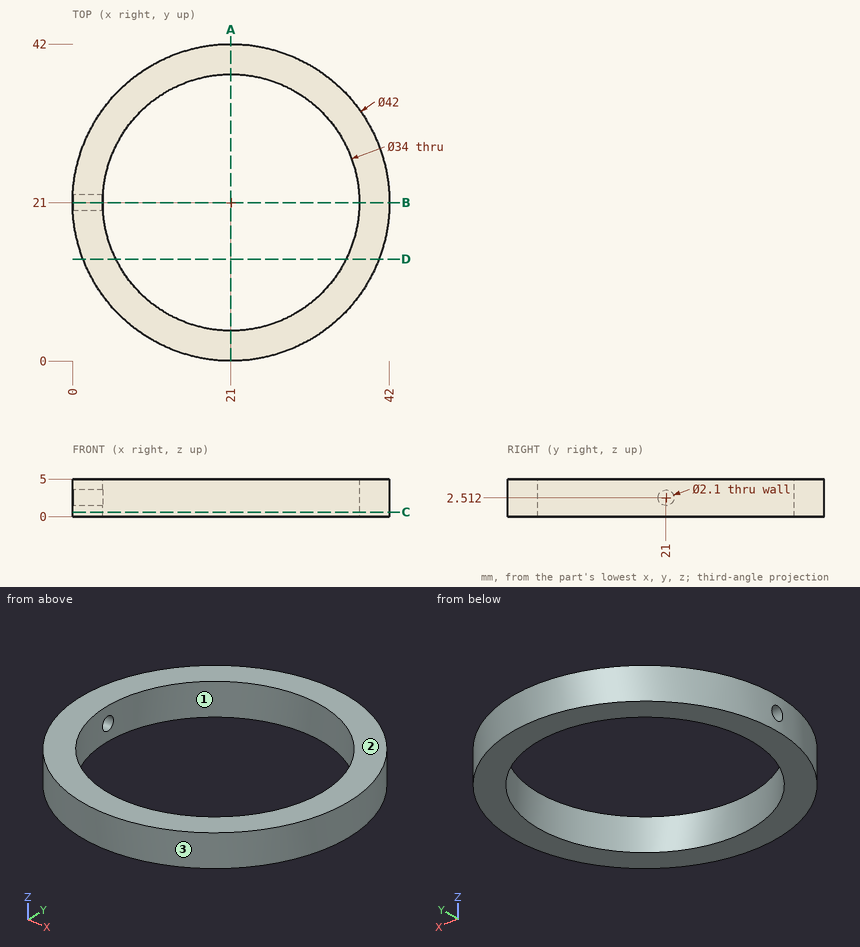
Design review of the part shown in the three views and the two pictorial views. Dimensions are in mm from the part's minimum x, y and z. Round coordinates to 2 decimals unless told otherwise and drop trailing zeros. Write each loop counter-clockwise with the first axis right and the second up, starting at its lowest first coordinate (ties: lowest second). Pieces come first, ordered by that corner, then holes. Notation, with made-up numbers: (2, 10.25) -> (38, 10.25) arc R11 ccw to (38, 17.25) -> close; hole circle Ø9 at (66.5, 83.5). An arc over 180 degrees is marked (long way). One line per question, with ' | ' between items. Start each with the question number.
1) Add section B-B (y = 21). Write out the cut boundary in (x, z).
2) For pin 1 Ø2.5 at (y, z) = (21, 2.51) entering from -X; pin 2 Ø2 at (y, z) = (34.5, 4) entering from -X (1 decimal); pin 3 Ø2 at (x, z) = (31.5, 0.5) entering from +Y, all flat-tipped, find the tip position at first contact; note any pin that passes through.
3) Add section A-A (x = 21). Write out the cut boundary in (y, z).
4) Wall thickness on line 1 along Y through (x, z) = (21, 3.55); line 2 along X through (y, z) = (31.5, 4.35); line 3 along Y through (x, z) = (18, 4.5) (1 decimal): over which ranges is each line inside the solid? List them lowest first.
5) Add section C-C (z = 0.6). Write out the cut boundary in (x, y).
6) Add section D-D (y = 13.5). Write out the cut boundary in (x, z) (3 decimals).
7) Mouldability with a two-part tool opening along Y and no side actions: class the marked faces 1, 2 and 3 as +Y half, -Y half, draft (parallel to the pull), parting line (faces both ways), or undercut.
Reported:
1) outline: (0, 0) -> (4, 0) -> (4, 1.46) -> (0, 1.46) -> close; (0, 3.56) -> (4, 3.56) -> (4, 5) -> (0, 5) -> close; (38, 0) -> (42, 0) -> (42, 5) -> (38, 5) -> close
2) pin 1: stops at x = 0 | pin 2: stops at x = 4.1 | pin 3: stops at y = 39.73
3) outline: (0, 0) -> (4, 0) -> (4, 5) -> (0, 5) -> close; (38, 0) -> (42, 0) -> (42, 5) -> (38, 5) -> close
4) line 1: y = 0 to 4, 38 to 42 | line 2: x = 2.81 to 7.63, 34.37 to 39.19 | line 3: y = 0.2 to 4.3, 37.7 to 41.8
5) outline: circle Ø42 at (21, 21); hole circle Ø34 at (21, 21)
6) outline: (1.385, 0) -> (5.744, 0) -> (5.744, 5) -> (1.385, 5) -> close; (36.256, 0) -> (40.615, 0) -> (40.615, 5) -> (36.256, 5) -> close
7) face 1: undercut | face 2: draft | face 3: parting line
